from build123d import *

# Parameters (mm, degrees)
BOSS_EXTRUDE1_DEPTH     = 98.552
BOSS_EXTRUDE2_DEPTH     = 32.004
SKETCH3_R               = 4.7625
CUT_EXTRUDE1_DEPTH      = 3.3114
FILLET1_R               = 12.7
SKETCH4_R               = 4.7625
CUT_EXTRUDE2_DEPTH      = 3.3114
SKETCH5_R               = 4.7625
CUT_EXTRUDE3_DEPTH      = 67.0146
CUT_EXTRUDE3_DEPTH_BACK = 3.3114
CUT_EXTRUDE4_REACH      = 79.809
SKETCH6_R               = 4.7625


with BuildPart() as part:
    # Sketch1 → Boss-Extrude1 (new body)
    with BuildSketch(Plane.XY):
        with BuildLine():
            Line((6.35, 0), (68.326, 0))
            Line((68.326, 0), (68.326, 2.3114))
            Line((68.326, 2.3114), (8.6614, 2.3114))
            ThreePointArc((8.6614, 2.3114), (4.171271939, 4.171271939), (2.3114, 8.6614))
            Line((2.3114, 8.6614), (2.3114, 58.010136575))
            ThreePointArc((2.3114, 58.010136575), (3.726523145, 62.006321058), (7.341160763, 64.22137384))
            Line((7.341160763, 64.22137384), (42.468530991, 71.687926876))
            Line((42.468530991, 71.687926876), (41.987963909, 73.94881724))
            Line((41.987963909, 73.94881724), (5.029760763, 66.093108654))
            ThreePointArc((5.029760763, 66.093108654), (1.415123145, 63.878055872), (0, 59.881871389))
            Line((0, 59.881871389), (0, 6.35))
            ThreePointArc((0, 6.35), (1.859871939, 1.859871939), (6.35, 0))
        make_face()
    extrude(amount=-BOSS_EXTRUDE1_DEPTH)

    # Sketch2 → Boss-Extrude2 (add)
    with BuildSketch(Plane(origin=(68.326, 0, 0), x_dir=(0, 0, -1), z_dir=(1, 0, 0))):
        with BuildLine():
            Line((98.552, 0), (133.35, 0))
            ThreePointArc((133.35, 0), (137.840128061, 1.859871939), (139.7, 6.35))
            Line((139.7, 6.35), (139.7, 53.34))
            Line((139.7, 53.34), (137.3886, 53.34))
            Line((137.3886, 53.34), (137.3886, 8.6614))
            ThreePointArc((137.3886, 8.6614), (135.528728061, 4.171271939), (131.0386, 2.3114))
            Line((131.0386, 2.3114), (98.552, 2.3114))
            Line((98.552, 2.3114), (98.552, 0))
        make_face()
    extrude(amount=-BOSS_EXTRUDE2_DEPTH)

    # Sketch3 → Cut-Extrude1 (cut, through all)
    with BuildSketch(Plane.XY.offset(-137.3886)):
        with BuildLine():
            Line((36.322, 53.34), (36.322, 37.338))
            ThreePointArc((36.322, 37.338), (41.008877287, 48.653122713), (52.324, 53.34))
            Line((52.324, 53.34), (36.322, 53.34))
        make_face()
        with BuildLine():
            ThreePointArc((52.324, 53.34), (63.639122713, 48.653122713), (68.326, 37.338))
            Line((68.326, 37.338), (68.326, 53.34))
            Line((68.326, 53.34), (52.324, 53.34))
        make_face()
        with Locations((52.324, 37.338)):
            Circle(SKETCH3_R)
    extrude(amount=-CUT_EXTRUDE1_DEPTH, mode=Mode.SUBTRACT)

    # Fillet1
    fillet1_edges = [part.edges().sort_by_distance(p)[0] for p in [
        (36.322, 1.1557, -98.552),
    ]]
    fillet(fillet1_edges, radius=FILLET1_R)

    # Sketch4 → Cut-Extrude2 (cut, through all)
    with BuildSketch(Plane(origin=(0, 2.3114, 0), x_dir=(1, 0, 0), z_dir=(0, 1, 0))):
        with Locations((48.514, 23.876)):
            Circle(SKETCH4_R)
        with Locations((48.514, 53.34)):
            Circle(SKETCH4_R)
        Polygon((52.451, 0), (68.326, 15.875), (68.326, 0), align=None)
    extrude(amount=-CUT_EXTRUDE2_DEPTH, mode=Mode.SUBTRACT)

    # Sketch5 → Cut-Extrude3 (cut, two sides)
    with BuildSketch(Plane(origin=(2.3114, 0, 0), x_dir=(0, 0, -1), z_dir=(1, 0, 0))) as cut_extrude3_sk:
        with Locations((17.526, 26.9494)):
            Circle(SKETCH5_R)
        with Locations((75.438, 26.9494)):
            Circle(SKETCH5_R)
        with Locations((17.526, 56.4134)):
            Circle(SKETCH5_R)
        with Locations((75.438, 56.4134)):
            Circle(SKETCH5_R)
    extrude(amount=CUT_EXTRUDE3_DEPTH, mode=Mode.SUBTRACT)
    extrude(cut_extrude3_sk.sketch, amount=-CUT_EXTRUDE3_DEPTH_BACK, mode=Mode.SUBTRACT)

    # Sketch6 → Cut-Extrude4 (cut, up to next)
    with BuildSketch(Plane(origin=(-13.22382174, 62.213189919, 0), x_dir=(0.978147601, 0.207911691, 0), z_dir=(-0.207911691, 0.978147601, 0)), mode=Mode.PRIVATE) as cut_extrude4_sk1:
        with Locations((34.855249784, 82.55)):
            Circle(SKETCH6_R)
    cut_extrude4_tool1 = extrude(cut_extrude4_sk1.sketch, amount=-CUT_EXTRUDE4_REACH, mode=Mode.PRIVATE) & part.part
    add(cut_extrude4_tool1.solids().sort_by_distance((20.869757, 69.460004, -82.55))[0], mode=Mode.SUBTRACT)
    # Sketch6 → Cut-Extrude4 (cut, up to next)
    with BuildSketch(Plane(origin=(-13.22382174, 62.213189919, 0), x_dir=(0.978147601, 0.207911691, 0), z_dir=(-0.207911691, 0.978147601, 0)), mode=Mode.PRIVATE) as cut_extrude4_sk2:
        with Locations((34.855249784, 19.05)):
            Circle(SKETCH6_R)
    cut_extrude4_tool2 = extrude(cut_extrude4_sk2.sketch, amount=-CUT_EXTRUDE4_REACH, mode=Mode.PRIVATE) & part.part
    add(cut_extrude4_tool2.solids().sort_by_distance((20.869757, 69.460004, -19.05))[0], mode=Mode.SUBTRACT)


solid = part.part
Build history of the part. All positions in model axes, mm. A direction names the side the tool comes from. Give positions to 0.01 mm unless a question says otherwise; leave off trailing zeros. Write each loop counter-clockwise with the first axis right and the second up, starting at its lowest first coordinate (ties: lowest second). Pieces come first, ordered by that corner, then holes. Notation, with made-up numbers: (-12, -4.5) - (37, -4.5) arc R23 ccw to (37, 26.5) - close; hole circle Ø1 at (61.25, -16). An arc over 180 degrees is marked (long way). Use one line per item in the form item = value. Start each with the question number.
1. Band-saw the part on D-D on y = 39. Write the cut outline in (x, z).
2. Band-saw the part on A-A on y = 12. Write the cut outline in (x, z).
3. Probe line 1 (Y direction, x = 54, z = -55.5); line 2 (Y direction, x = 41, z = -76.5). List the from-to ranges inside material, lowest first. Write a range as [from, to].
4. Two-plate mould, pull along Z, no slides. Class faces 5 (the face through (1.17, 27.16, -70.68)), 6 (the face through (2.311, 33, -49)), 7 (the face through (1, 32, 0)): released by +Z, released by -Z, zero draft, split by the parting line, or undercut.
5. Band-saw the part on B-B on z = -53.34. Write the cut outline in (x, y), plus the area to 3 significant figures.
6. Band-saw the part on C-C on x = 12.5. Write the cut outline in (y, z).
7. Drop flat-ended pins along their axis: pin 1 Ø12 at (x, z) = (50, -23) entering from +Y; pin 2 Ø5.5 at (x, z) = (48.514, -53.34) entering from +Y; pin 3 Ø24.5 at (y, z) = (37, -41) entering from +X; pin 4 Ø10 at (x, z) = (16, -19) entering from +Y. Give the stop position or say it passes through.
8. 3-axis set-ups, long thin cutter, end or side, ignore diameter. For faces 1 (the face through (3.69, 61.96, -48.59)), 2 (the face through (53, 31, -137.389)), 3 (the face through (36.322, 10, -138)), 4 (the face through (53, 30, -139.7)): which of +Z, -Z, +X, -X, +Y, -Y reach the whole face in a straight line?
Conclusion:
q1.outline = (0, -98.55) - (2.31, -98.55) - (2.31, 0) - (0, 0) - close; (36.41, -139.7) - (47.86, -139.7) - (47.86, -137.39) - (36.41, -137.39) - close; (56.79, -139.7) - (68.24, -139.7) - (68.24, -137.39) - (56.79, -137.39) - close
q2.outline = (0, -98.55) - (2.31, -98.55) - (2.31, 0) - (0, 0) - close; (36.32, -139.7) - (68.33, -139.7) - (68.33, -137.39) - (36.32, -137.39) - close
q3.line_1 = [0, 2.31]
q3.line_2 = [0, 2.31], [71.38, 73.74]
q4.face_5 = undercut
q4.face_6 = zero draft
q4.face_7 = released by +Z
q5.outline = (0, 6.35) arc R6.35 ccw to (6.35, 0) - (43.75, 0) - (43.75, 2.31) - (8.66, 2.31) arc R6.35 cw to (2.31, 8.66) - (2.31, 58.01) arc R6.35 cw to (7.34, 64.22) - (42.47, 71.69) - (41.99, 73.95) - (5.03, 66.09) arc R6.35 ccw to (0, 59.88) - close; (53.28, 0) - (68.33, 0) - (68.33, 2.31) - (53.28, 2.31) - close
q5.area = 376 mm²
q6.outline = (0, -98.55) - (2.31, -98.55) - (2.31, 0) - (0, 0) - close; (65.32, -98.55) - (67.68, -98.55) - (67.68, 0) - (65.32, 0) - close
q7.pin_1 = 2.31
q7.pin_2 = through
q7.pin_3 = 2.31
q7.pin_4 = 69.01
q8.face_1 = +Z, -Z, +X
q8.face_2 = +Z, +X, -X, +Y
q8.face_3 = -Z, -X, +Y, -Y
q8.face_4 = -Z, +X, -X, +Y, -Y
